```python
from build123d import *

# Parameters (mm, degrees)
SKETCH_R     = 6.1
SKETCH_R_2   = 8.1
PAD_DEPTH    = 10
CHAMFER_SIZE = 0.5


with BuildPart() as part:
    # Sketch → Pad (new body)
    with BuildSketch(Plane.XY):
        with BuildLine():
            ThreePointArc((-60, 15), (-75, 0), (-60, -15))
            Line((-60, -15), (60, -15))
            ThreePointArc((60, -15), (75, 0), (60, 15))
            Line((-60, 15), (60, 15))
        make_face()
        with Locations((60, 0)):
            Circle(SKETCH_R, mode=Mode.SUBTRACT)
        with Locations((-60, 0)):
            Circle(SKETCH_R_2, mode=Mode.SUBTRACT)
    extrude(amount=PAD_DEPTH)

    # Chamfer
    chamfer_edges = [part.edges().sort_by_distance(p)[0] for p in [
        (53.9, 0, 10),
        (-68.1, 0, 10),
        (53.9, 0, 0),
        (-68.1, 0, 0),
    ]]
    chamfer(chamfer_edges, length=CHAMFER_SIZE)


solid = part.part
```
Verification items for the finished model (mm, model axes). Coordinates: 2 decimals unless noted, no trailing zeros. Loops run counter-clockwise (first coordinate to the right, second up) from the corner with the lowest first, then second, coordinate; pieces in that order, holes last. Notation, with made-up numbers: (2.5, 51) -> (16.5, 51) arc R38 ccw to (16.5, 89) -> close; hole circle Ø9 at (57.5, -1). An arc over 180 degrees is marked (long way). Put each result on its own line as item: value.
1. Section check C-C, the plane y = 10. Record the boundary of the cut face in (x, z).
Result set:
outline: (-71.18, 0) -> (71.18, 0) -> (71.18, 10) -> (-71.18, 10) -> close
2. Thickness scan on line 1 (Y direction, x = 60, z = 6.75); line 2 (Y direction, x = -60, z = 3.5); line 3 (X direction, y = -1, z = 6.75). Record the ranges inside material, lowest first.
Result set:
line 1: y = -15 to -6.1, 6.1 to 15
line 2: y = -15 to -8.1, 8.1 to 15
line 3: x = -74.97 to -68.04, -51.96 to 53.98, 66.02 to 74.97
3. Gauge pin test, flat ends, axial feed: P1, Ø2, axis at y = 9.5, z = 5.5, coming from the -X side; P2, Ø6, axis at y = 8.5, z = 9, coming from the -X side. Record the tip position at first contact, or that the pin passes through.
Result set:
P1: stops at x = -72.36
P2: stops at x = -73.96
4. Section check D-D, the plane y = -11.5. Record the boundary of the cut face in (x, z).
Result set:
outline: (-69.63, 0) -> (69.63, 0) -> (69.63, 10) -> (-69.63, 10) -> close
5. Mould release check, pull along X, two halves, no side actions. Record for faces 1 (the face through (-75, 0, 5)), 2 (the face through (65.635, -2.336, 4.937)), 3 (the face through (-1, 0, 10)): pulls with the +X half, pulls with the -X half, needs draft (parallel to the pull), parting line crosses it, or undercut.
Result set:
face 1: pulls with the -X half
face 2: undercut
face 3: needs draft
6. Section check A-A, the plane y = 0. Record the boundary of the cut face in (x, z), then the cut area to 4 significant figures.
Result set:
outline: (-75, 0) -> (-68.6, 0) -> (-68.1, 0.5) -> (-68.1, 9.5) -> (-68.6, 10) -> (-75, 10) -> close; (-51.9, 0.5) -> (-51.4, 0) -> (53.4, 0) -> (53.9, 0.5) -> (53.9, 9.5) -> (53.4, 10) -> (-51.4, 10) -> (-51.9, 9.5) -> close; (66.1, 0.5) -> (66.6, 0) -> (75, 0) -> (75, 10) -> (66.6, 10) -> (66.1, 9.5) -> close
area: 1,215 mm^2
7. Section check B-B, the plane z = 6.75. Record the boundary of the cut face in (x, y), then the cut area to 3 significant figures.
Result set:
outline: (-60, -15) -> (60, -15) arc R15 ccw to (60, 15) -> (-60, 15) arc R15 ccw to start; hole circle Ø16.2 at (-60, 0); hole circle Ø12.2 at (60, 0)
area: 3,980 mm^2
